from build123d import *

# Parameters (mm, degrees)
AUFSATZ_LINEAR_AUSTRAGEN1_DEPTH             = 3
FORMSENKUNG_F_R_M4_SENKSCHRAUBE_MIT_2_COUNT = 2
FORMSENKUNG_F_R_M4_SENKSCHRAUBE_MIT_2_PITCH = 284
FORMSENKUNG_F_R_M4_SENKSCHRAUBE_MIT_3_COUNT = 2
FORMSENKUNG_F_R_M4_SENKSCHRAUBE_MIT_3_PITCH = 268.942837793
FORMSENKUNG_F_R_M4_SENKSCHRAUBE_MIT_4_COUNT = 2
FORMSENKUNG_F_R_M4_SENKSCHRAUBE_MIT_4_PITCH = 374.441250399
SKIZZE4_R                                   = 95
SCHNITT_LINEAR_AUSTRAGEN1_DEPTH             = 10


with BuildPart() as part:
    # Skizze1 → Aufsatz-Linear austragen1 (new body)
    with BuildSketch(Plane.XY):
        Polygon((15.000749991, 0), (15.000749991, -300), (38.000749991, -300), (38.000749991, -277), (302.000749991, -277), (302.000749991, -23), (38.000749991, -23), (38.000749991, 0), align=None)
    extrude(amount=AUFSATZ_LINEAR_AUSTRAGEN1_DEPTH)

    # Skizze3 → Formsenkung für M4 Senkschraube mit Innensechskant1 (revolve, cut)
    with BuildSketch(Plane(origin=(26.500749991, -8, 3), x_dir=(0, -1, 0), z_dir=(1, 0, 0))):
        Polygon((0, 0), (0, 3), (2.25, 3), (2.25, 2.34), (4.59, 0), align=None)
    formsenkung_f_r_m4_senkschraube_mit_inne = revolve(axis=Axis((26.500749991, -8, 9.35), (0, 0, -1)), mode=Mode.SUBTRACT)

    # Formsenkung f_r M4 Senkschraube mit  2: Formsenkung für M4 Senkschraube mit Innensechskant1 ×2
    with Locations(*[(0, -i * FORMSENKUNG_F_R_M4_SENKSCHRAUBE_MIT_2_PITCH, 0) for i in range(1, FORMSENKUNG_F_R_M4_SENKSCHRAUBE_MIT_2_COUNT)]):
        add(formsenkung_f_r_m4_senkschraube_mit_inne, mode=Mode.SUBTRACT)

    # Formsenkung f_r M4 Senkschraube mit  3: Formsenkung für M4 Senkschraube mit Innensechskant1 ×2
    with Locations(*[Vector(0.9964942818315755, -0.08366090052690477, 0) * (i * FORMSENKUNG_F_R_M4_SENKSCHRAUBE_MIT_3_PITCH) for i in range(1, FORMSENKUNG_F_R_M4_SENKSCHRAUBE_MIT_3_COUNT)]):
        add(formsenkung_f_r_m4_senkschraube_mit_inne, mode=Mode.SUBTRACT)

    # Formsenkung f_r M4 Senkschraube mit  4: Formsenkung für M4 Senkschraube mit Innensechskant1 ×2
    with Locations(*[Vector(0.7157331082373348, -0.6983739097166529, 0) * (i * FORMSENKUNG_F_R_M4_SENKSCHRAUBE_MIT_4_PITCH) for i in range(1, FORMSENKUNG_F_R_M4_SENKSCHRAUBE_MIT_4_COUNT)]):
        add(formsenkung_f_r_m4_senkschraube_mit_inne, mode=Mode.SUBTRACT)

    # Skizze4 → Schnitt-Linear austragen1 (cut)
    with BuildSketch(Plane.XY.offset(3)):
        with Locations((127.000749991, -150)):
            Circle(SKIZZE4_R)
    extrude(amount=-SCHNITT_LINEAR_AUSTRAGEN1_DEPTH, mode=Mode.SUBTRACT)


solid = part.part
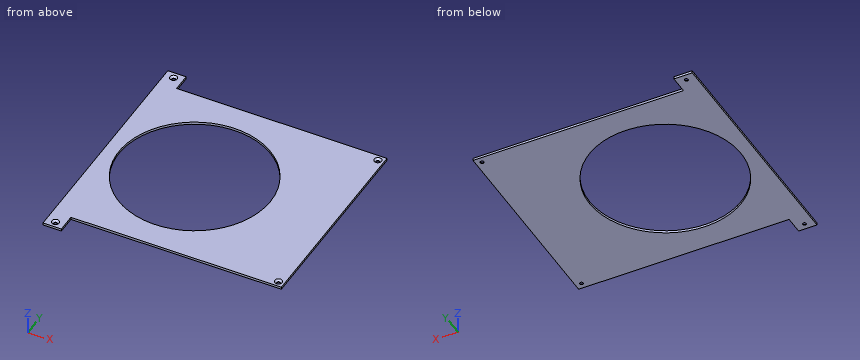
Model file for the job. Use its own axes, mm. Give positions to 0.01 mm unless a question says otherwise; leave off trailing zeros. Loops run counter-clockwise (first coordinate to the right, second up) from the corner with the lowest first, then second, coordinate; pieces in that order, holes last.
1) Flat gauge pins, fed straight in: pin 1 Ø6 at (x, y) = (294.5, -269.5) entering from +Z; pin 2 Ø1.5 at (x, z) = (107.5, 1) entering from +Y; pin 3 Ø0.9 at (y, z) = (-16.5, 1) entering from +X. Where does each tip first touch, or does it go through?
2) Saw through at A-A (y = -150). Write the cut outline in (x, z), plus the area to 3 significant figures.
3) Saw through at B-B (z = 1.9). Write the cut outline in (x, y).
4) Wall check: line 1 (X direction, y = -30.5, z = 0.35); line 2 (X direction, y = -8, z = 0.45); line 3 (Y direction, x = 106, z = 0.25). Give the ranges that are in metal, low to high.
5) Saw through at C-C (x = 99). Write the cut outline in (y, z), plus the area to 3 significant figures.
Answer block:
1. pin 1: stops at z = 1.41
1. pin 2: stops at y = -23
1. pin 3: stops at x = 38
2. outline: (15, 0) - (32, 0) - (32, 3) - (15, 3) - close; (222, 0) - (302, 0) - (302, 3) - (222, 3) - close
2. area: 291 mm2
3. outline: (15, -300) - (38, -300) - (38, -277) - (302, -277) - (302, -23) - (38, -23) - (38, 0) - (15, 0) - close; hole circle Ø6.98 at (26.5, -292); hole circle Ø6.98 at (26.5, -8); hole circle Ø190 at (127, -150); hole circle Ø6.98 at (294.5, -269.5); hole circle Ø6.98 at (294.5, -30.5)
4. line 1: x = 15 to 292.25, 296.75 to 302
4. line 2: x = 15 to 24.25, 28.75 to 38
4. line 3: y = -277 to -242.65, -57.35 to -23
5. outline: (-277, 0) - (-240.78, 0) - (-240.78, 3) - (-277, 3) - close; (-59.22, 0) - (-23, 0) - (-23, 3) - (-59.22, 3) - close
5. area: 217 mm2
